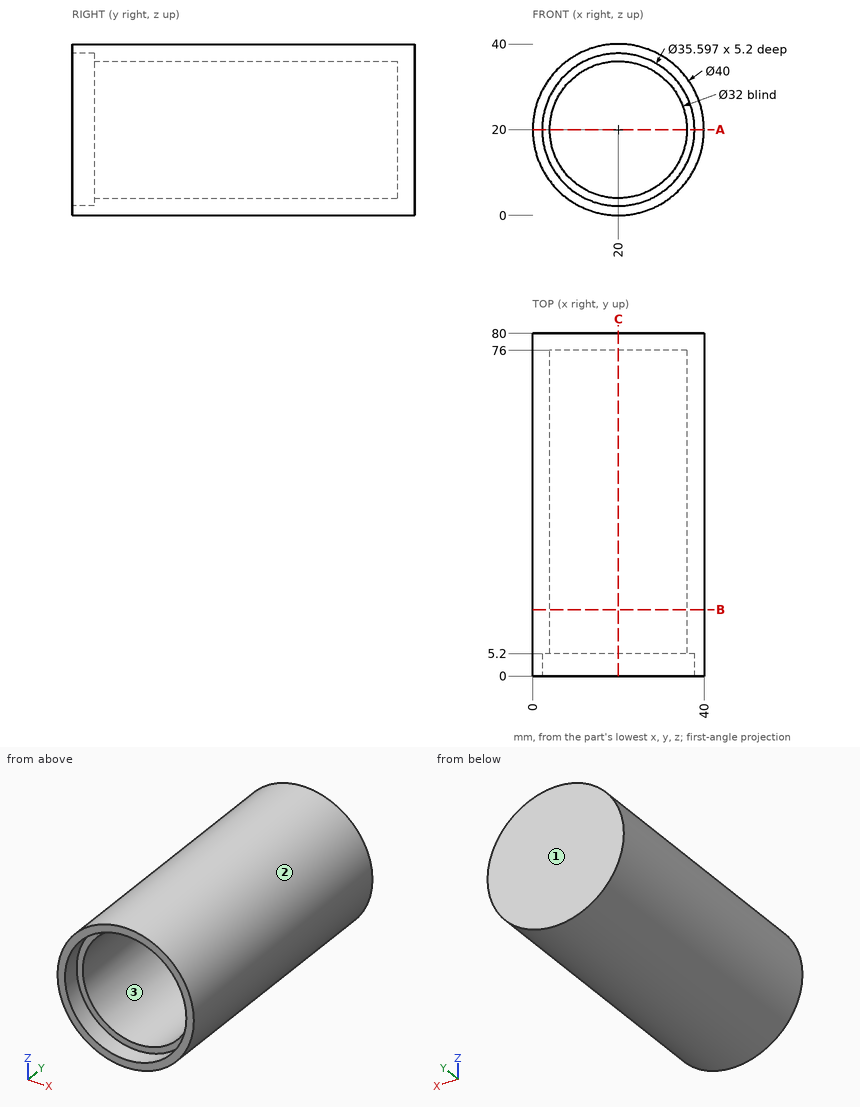
For this review, use the dimensioned drawing (mm, ordinates from the lowest corner) and the shaded views. Coordinates: 2 decimals unless noted, no trailing zeros. Order: outer loops, then holes, each group sorted by start corner. A loop starts at its lowest first (then second) coordinate and runs counter-clockwise, first axis right, second up. Notation, with made-up numbers: M -15,73 L 38,73 A26 ccw 38,103 Z; hole C 60,38.25 d10. An arc over 180 degrees is marked long. Answer as a JSON object with one key per item and string values. Group by question number.
1) Add section B-B, the plane y = 15.5. Write out the cut boundary in (x, z), then the cut area to 3 significant figures.
2) Wall thickness on L1, parallel to Z at x = 20, y = 40; L2, parallel to Z at x = 20, y = 3; L3, parallel to Y at x = 8.5, z = 31: over which ranges is each line inside the solid? List them lowest first.
3) Add section C-C, the plane x = 20. Write out the cut boundary in (y, z), then the cut area to 3 significant figures.
4) Add section A-A, the plane z = 20. Write out the cut boundary in (x, y), then the cut area to 3 significant figures.
5) Mouldability with a two-part tool opening along X and no side actions: class the marked faces 1, 2 and 3 as pulls with the +X half, pulls with the -X half, needs draft (parallel to the pull), parting line crosses it, or undercut.
6) For pin 1 (1 mm diameter, centred on x = 18, y = 66, fed in from +Z); pin 2 (3 mm diameter, centred on x = 24, y = 43.5, fed in from +Z); pin 3 (16 mm diameter, centred on x = 19.5, z = 23, fed in from -Y), all flat-tipped, find the tip position at first contact; note any pin that passes through.
Computed values:
{
 "1": {"outline": "C 20,20 d40; hole C 20,20 d32", "area": "452 mm^2"},
 "2": {"L1": "z = 0 to 4, 36 to 40", "L2": "z = 0 to 2.2, 37.8 to 40", "L3": "y = 76 to 80"},
 "3": {"outline": "M 0,0 L 80,0 L 80,40 L 0,40 L 0,37.8 L 5.2,37.8 L 5.2,36 L 76,36 L 76,4 L 5.2,4 L 5.2,2.2 L 0,2.2 Z", "area": "749 mm^2"},
 "4": {"outline": "M 0,0 L 2.2,0 L 2.2,5.2 L 4,5.2 L 4,76 L 36,76 L 36,5.2 L 37.8,5.2 L 37.8,0 L 40,0 L 40,80 L 0,80 Z", "area": "749 mm^2"},
 "5": {"face 1": "needs draft", "face 2": "parting line crosses it", "face 3": "undercut"},
 "6": {"pin 1": "stops at z = 39.94", "pin 2": "stops at z = 39.84", "pin 3": "stops at y = 76"}
}
